Can you work these out from the model? Positions are in its coordinate system, mm. Coordinates: 2 decimals unless noted, no trailing zeros. Loops run counter-clockwise (first coordinate to the right, second up) from the corner with the lowest first, then second, coordinate; pieces in that order, holes last. Notation, with made-up numbers: (-22, -15) -> (-1, -15) arc R18 cw to (-1, -3) -> close; hole circle Ø6 at (43, -22). An arc over 180 degrees is marked (long way). Use one line per item in the form item = value. Start each with the question number.
(1) Imagine slicing it at A-A (y = 3). List the corners of the cut face in (x, z) for me.
(2) Imagine slicing it at C-C (z = 0.35). State how many separate pieces and enclosed holes the cut face has, plus the area to 3 significant figures.
(3) I'm going to push a flat-ended pin straight in: pin 1 (0.6 mm diameter, centred on y = 0, z = 0.5, fed in from +X). Where does the tip first touch, or does it pass through?
(4) I need wall thicknesses on line 1 (Y direction, x = 0.5, z = 0.8); line 2 (X direction, y = 5, z = 0.6); line 3 (Y direction, x = 0.75, z = 1). Which ranges of each line are inside material? Lowest first, please. Write a range as [from, to].
(5) Imagine slicing it at D-D (x = -8). List the corners of the cut face in (y, z) for me, plus the area to 3 significant figures.
(6) Imagine slicing it at B-B (x = 2). List the corners of the cut face in (y, z) for me, plus the area to 3 significant figures.
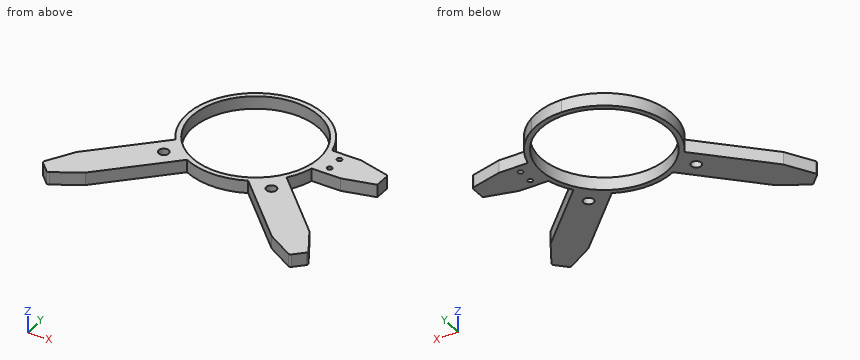
Autodesk Inventor part; units mm, degrees
ref_plane "YZ Plane" through (0, 0, 0) normal (1, 0, 0) x (0, 1, 0)
ref_plane "XZ Plane" through (0, 0, 0) normal (0, 1, 0) x (-1, 0, 0)
ref_plane "XY Plane" through (0, 0, 0) normal (0, 0, 1) x (1, 0, 0)
sketch "Sketch1" plane through (0, 0, 0) normal (0, 0, 1) x (1, 0, 0)
  line L0 (-0.0012, 9.6891) -> (-0.0012, -0.0155) construction
  circle A0 centre (-0.0012, -0.0155) radius 6.35
  line L1 (9.3601, -12.4316) -> (3.0739, -6.1454)
  line L2 (5.5879, -3.9897) -> (11.6952, -10.0969)
  line L3 (9.3601, -12.4316) -> (12.1799, -14.1019)
  line L4 (12.1799, -14.1019) -> (13.3653, -12.9165)
  line L5 (13.3653, -12.9165) -> (11.6952, -10.0969)
  line L6 (13.4673, -0.0155) -> (-6.3512, -0.0155) construction
  arc A1 (-3.0764, -6.1454) -> (3.0739, -6.1454) centre (-0.0012, -0.0155) ccw
  arc A2 (0.9828, -6.8026) -> (3.0739, -6.1454) centre (-0.0012, -0.0155) ccw
  arc A3 (-0.0012, 6.8425) -> (-5.5904, -3.9897) centre (-0.0012, -0.0155) ccw
  arc A4 (-6.8132, -0.8093) -> (-5.5904, -3.9897) centre (-0.0012, -0.0155) ccw
  arc A5 (5.5879, -3.9897) -> (6.6536, -1.6723) centre (-0.0012, -0.0155) ccw
  arc A6 (6.6536, 1.6412) -> (3.738, 5.7334) centre (-0.0012, -0.0155) ccw
  arc A7 (5.5879, -3.9897) -> (6.6536, -1.6723) centre (-0.0012, -0.0155) ccw
  arc A8 (6.6536, 1.6412) -> (-0.0012, 6.8425) centre (-0.0012, -0.0155) ccw
  line L7 (5.5879, -3.9897) -> (21.5848, -3.9897) construction
  line L8 (-9.3626, -12.4316) -> (-3.0764, -6.1454)
  line L9 (-5.5904, -3.9897) -> (-11.6977, -10.0969)
  line L10 (-9.3626, -12.4316) -> (-12.1824, -14.1019)
  line L11 (-12.1824, -14.1019) -> (-13.3678, -12.9165)
  line L12 (-13.3678, -12.9165) -> (-11.6977, -10.0969)
  line L13 (9.5746, 1.6412) -> (12.7483, 0.8287)
  line L14 (6.6536, 1.6412) -> (9.5746, 1.6412)
  line L15 (9.5746, -1.6723) -> (12.7483, -0.8598)
  line L16 (6.6536, -1.6723) -> (9.5746, -1.6723)
  circle A9 centre (7.9363, -0.8093) radius 0.254
  circle A10 centre (7.9363, 0.7782) radius 0.254
  circle A11 centre (-5.4113, -6.1454) radius 0.508
  line L17 (12.7483, 0.8287) -> (12.7483, -0.8598)
  circle A12 centre (5.4088, -6.1454) radius 0.508
  point P0 (13.4229, -0.6871)
  point P1 (13.4673, -0.0008)
  dimension "d35" = 12.7
  dimension "d72" = 8.89
  dimension "d73" = 3.2774
  dimension "d77" = 194.36
  dimension "d78" = 1.6764
  dimension "d115" = 90
  dimension "d128" = 165.64
  dimension "d148" = 0.508
  dimension "d154" = 3.302
  dimension "d160" = 3.276
  dimension "d166" = 0.508
  dimension "d168" = 7.9375
  dimension "d169" = 0.863
  dimension "d176" = 1.016
  dimension "d182" = 3.3135
  dimension "d184" = 1.6885
  dimension "d191" = 2.921
  dimension "d234" = 24.3623
extrude "Extrusion8" add sketch "Sketch1" along normal blind 1.27
fillet "Fillet57" radius 0.254 1 edges at (-12.1824, -14.1019, 0.635)
fillet "Fillet58" radius 0.254 1 edges at (-13.3678, -12.9165, 0.635)
fillet "Fillet59" radius 0.254 1 edges at (13.3653, -12.9165, 0.635)
fillet "Fillet60" radius 0.254 1 edges at (12.1799, -14.1019, 0.635)
fillet "Fillet63" radius 0.254 1 edges at (12.7483, 0.8287, 0.635)
equation "\"BendRadius\" = Thickness"
equation "\"BendReliefWidth\" = Thickness"
equation "\"BendReliefDepth\" = 0.5 * Thickness"
equation "\"CornerReliefSize\" = 4 * Thickness"
equation "\"MinimumRemnant\" = 2 * Thickness"
equation "\"TransitionRadius\" = BendRadius"
equation "\"JacobiRadiusSize\" = BendRadius"
equation "\"GapSize\" = Thickness"
properties part number "CircularHeadbar_large_simple"
Worked out:
q1.outline = (-6.16, 0) -> (-5.59, 0) -> (-5.59, 1.27) -> (-6.16, 1.27) -> close; (5.59, 0) -> (6.16, 0) -> (6.16, 1.27) -> (5.59, 1.27) -> close
q2.separate_pieces = 1
q2.enclosed_holes = 5
q2.area = 109 mm2
q3.pin_1 = 12.75
q4.line_1 = [-6.86, -6.35], [6.31, 6.82]
q4.line_2 = [-4.68, -3.9], [3.89, 4.68]
q4.line_3 = [-6.83, -6.32], [6.29, 6.8]
q5.outline = (-11.07, 0) -> (-6.4, 0) -> (-6.4, 1.27) -> (-11.07, 1.27) -> close
q5.area = 5.93 mm2
q6.outline = (-6.58, 0) -> (-6.04, 0) -> (-6.04, 1.27) -> (-6.58, 1.27) -> close; (6.01, 0) -> (6.54, 0) -> (6.54, 1.27) -> (6.01, 1.27) -> close
q6.area = 1.35 mm2
